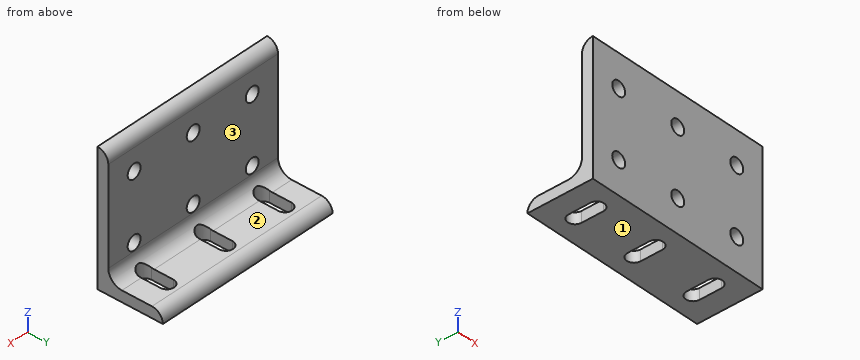
Solid Edge part; units mm, degrees
sketch "Sketch1" plane through (0, 0, 0) normal (1, 0, 0) x (0, 1, 0)
  line L0 (0, 76.2) -> (0, 0)
  line L1 (0, 0) -> (38.1, 0)
  arc A0 (38.1, 0) -> (31.75, 6.35) centre (31.75, 0) ccw
  line L2 (31.75, 6.35) -> (14.2748, 6.35)
  arc A1 (14.2748, 6.35) -> (6.35, 14.2748) centre (14.2748, 14.2748) cw
  line L3 (6.35, 14.2748) -> (6.35, 69.85)
  arc A2 (6.35, 69.85) -> (0, 76.2) centre (0, 69.85) ccw
extrude "ExtrudedProtrusion_1" add sketch "Sketch1" against normal blind 54.7624 and the other way blind 54.7624
hole "Hole_1" at (38.1, 0, 19.05) direction (0, 1, 0) diameter 8.3312 depth 6.985
hole "Hole_2" at (0, 0, 19.05) direction (0, 1, 0) diameter 8.3312 depth 6.985
hole "Hole_3" at (-38.1, 0, 19.05) direction (0, 1, 0) diameter 8.3312 depth 6.985
hole "Hole_4" at (38.1, 0, 57.15) direction (0, 1, 0) diameter 8.3312 depth 6.985
hole "Hole_5" at (0, 0, 57.15) direction (0, 1, 0) diameter 8.3312 depth 6.985
hole "Hole_6" at (-38.1, 0, 57.15) direction (0, 1, 0) diameter 8.3312 depth 6.985
sketch "Sketch2" plane through (0, 0, 0) normal (0, 0, 1) x (1, 0, 0)
  arc A0 (33.9344, 12.7) -> (42.2656, 12.7) centre (38.1, 12.7) ccw
  line L0 (42.2656, 12.7) -> (42.2656, 25.4)
  arc A1 (42.2656, 25.4) -> (33.9344, 25.4) centre (38.1, 25.4) ccw
  line L1 (33.9344, 25.4) -> (33.9344, 12.7)
extrude "ExtrudedCutout_1" cut sketch "Sketch2" along normal blind 9.525
sketch "Sketch3" plane through (0, 0, 0) normal (0, 0, 1) x (1, 0, 0)
  arc A0 (-4.1656, 12.7) -> (4.1656, 12.7) centre (0, 12.7) ccw
  line L0 (4.1656, 12.7) -> (4.1656, 25.4)
  arc A1 (4.1656, 25.4) -> (-4.1656, 25.4) centre (0, 25.4) ccw
  line L1 (-4.1656, 25.4) -> (-4.1656, 12.7)
extrude "ExtrudedCutout_2" cut sketch "Sketch3" along normal blind 9.525
sketch "Sketch4" plane through (0, 0, 0) normal (0, 0, 1) x (1, 0, 0)
  arc A0 (-42.2656, 12.7) -> (-33.9344, 12.7) centre (-38.1, 12.7) ccw
  line L0 (-33.9344, 12.7) -> (-33.9344, 25.4)
  arc A1 (-33.9344, 25.4) -> (-42.2656, 25.4) centre (-38.1, 25.4) ccw
  line L1 (-42.2656, 25.4) -> (-42.2656, 12.7)
extrude "ExtrudedCutout_3" cut sketch "Sketch4" along normal blind 9.525
properties part number "4281"
Build history of the part. All positions in model axes, mm. Face numbers are marked on the shaded views. Coordinates: 2 decimals unless noted, no trailing zeros. Order: outer loops, then holes, each group sorted by start corner. A loop starts at its lowest first (then second) coordinate and runs counter-clockwise, first axis right, second up. Notation, with made-up numbers: (-29.75, -7.75) -> (-10.75, -7.75) arc R15 ccw to (-10.75, -0.75) -> close; hole circle Ø10 at (-23.75, 25.25). An arc over 180 degrees is marked (long way). Answer in a Markdown table with one row per item. Add a question column.
Q1. Band-saw the part on A-A, the plane x = 0. List the corners of the cut face in (y, z).
Q2. Mould opens along Z. For the marked faces 1, 2 and 3 say: +Z half, -Z half, draft (parallel to the pull), parting line (faces both ways), or undercut.
Q3. Drop flat-ended pins along their axis: pin 1 (11 mm diameter, centred on x = -38.1, z = 19.05, fed in from +Y); pin 2 (1 mm diameter, centred on x = -4.5, z = 21.5, fed in from +Y); pin 3 (7.5 mm diameter, centred on x = 0, z = 19.05, fed in from -Y); pin 4 (19 mm diameter, centred on x = 24.5, y = 20.5, fed in from +Z). Give the stop position or say it passes through.
Q4. Band-saw the part on D-D, the plane z = 30. List the corners of the cut face in (x, y).
Q5. Wall check: line 1 along X through (y, z) = (5, 57); line 2 along Z through (x, y) = (0, 5); line 3 along Z through (x, y) = (0, 3). Give the ranges that are in metal, low to high. Write a range as [from, to].
Q6. Band-saw the part on C-C, the plane x = 27.5. List the corners of the cut face in (y, z).
Q7. Band-saw the part on B-B, the plane z = 19.05. List the corners of the cut face in (x, y), then the cut area to 3 significant figures.
Answers follow:
| question | item | result |
|---|---|---|
| 1 | outline | (0, 0) -> (8.53, 0) -> (8.53, 8.81) arc R7.92 cw to (6.35, 14.27) -> (6.35, 14.88) -> (0, 14.88) -> close; (0, 23.22) -> (6.35, 23.22) -> (6.35, 52.98) -> (0, 52.98) -> close; (0, 61.32) -> (6.35, 61.32) -> (6.35, 69.85) arc R6.35 ccw to (0, 76.2) -> close; (29.57, 0) -> (38.1, 0) arc R6.35 ccw to (31.75, 6.35) -> (29.57, 6.35) -> close |
| 2 | face 1 | -Z half |
| 2 | face 2 | +Z half |
| 2 | face 3 | draft |
| 3 | pin 1 | y = 6.38 |
| 3 | pin 2 | y = 6.35 |
| 3 | pin 3 | through |
| 3 | pin 4 | z = 7.06 |
| 4 | outline | (-54.76, 0) -> (54.76, 0) -> (54.76, 6.35) -> (-54.76, 6.35) -> close |
| 5 | line 1 | [-54.76, -42.26], [-33.94, -4.16], [4.16, 33.94], [42.26, 54.76] |
| 5 | line 2 | [0, 14.88], [23.22, 52.98], [61.32, 73.76] |
| 5 | line 3 | [0, 14.88], [23.22, 52.98], [61.32, 75.45] |
| 6 | outline | (0, 0) -> (38.1, 0) arc R6.35 ccw to (31.75, 6.35) -> (14.27, 6.35) arc R7.92 cw to (6.35, 14.27) -> (6.35, 69.85) arc R6.35 ccw to (0, 76.2) -> close |
| 7 | outline | (-54.76, 0) -> (-42.27, 0) -> (-42.27, 6.35) -> (-54.76, 6.35) -> close; (-33.93, 0) -> (-4.17, 0) -> (-4.17, 6.35) -> (-33.93, 6.35) -> close; (4.17, 0) -> (33.93, 0) -> (33.93, 6.35) -> (4.17, 6.35) -> close; (42.27, 0) -> (54.76, 0) -> (54.76, 6.35) -> (42.27, 6.35) -> close |
| 7 | area | 537 mm^2 |
